Verification items for the finished model (mm, model axes). Face numbers are marked on the shaded views. A direction names the side the tool comes from. Round coordinates to 2 decimals unless told otherwise and drop trailing zeros. Write each loop counter-clockwise with the first axis right and the second up, starting at its lowest first coordinate (ties: lowest second). Pieces come first, ordered by that corner, then holes. Notation, with made-up numbers: (-15, -38.5) - (26, -38.5) arc R30 ccw to (26, -8.5) - close; hole circle Ø8 at (31, 19.25). An arc over 180 degrees is marked (long way). Answer as a JSON object with one key per item and string values.
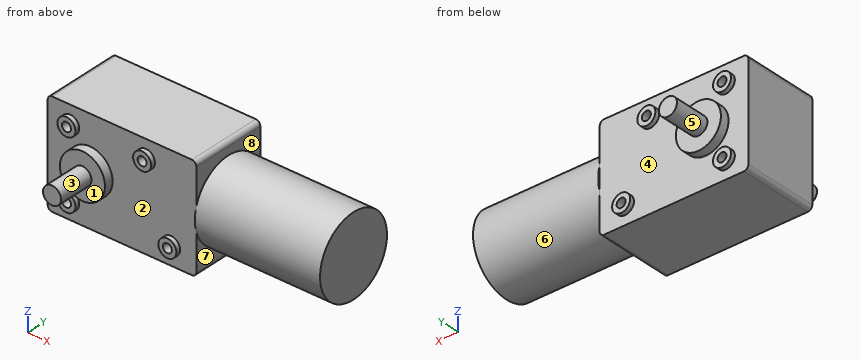
```python
from build123d import *

# Parameters (mm, degrees)
BOSS_EXTRUDE1_DEPTH = 21
SKETCH2_R           = 5
BOSS_EXTRUDE2_DEPTH = 2.5
SKETCH3_R           = 2.5
CUT_EXTRUDE1_DEPTH  = 6
SKETCH6_R           = 12.5
BOSS_EXTRUDE5_DEPTH = 5
SKETCH4_R           = 5
BOSS_EXTRUDE3_DEPTH = 20
SKETCH5_R           = 22
BOSS_EXTRUDE4_DEPTH = 69.5


with BuildPart() as part:
    # Sketch1 → Boss-Extrude1 (new, symmetric)
    with BuildSketch(Plane(origin=(0, 0, 0), x_dir=(1, 0, 0), z_dir=(0, 1, 0))):
        with BuildLine():
            Line((-38.75, -29), (38.75, -29))
            ThreePointArc((38.75, -29), (40.517766953, -28.267766953), (41.25, -26.5))
            Line((41.25, -26.5), (41.25, 26.5))
            ThreePointArc((41.25, 26.5), (40.517766953, 28.267766953), (38.75, 29))
            Line((38.75, 29), (-38.75, 29))
            ThreePointArc((-38.75, 29), (-40.517766953, 28.267766953), (-41.25, 26.5))
            Line((-41.25, 26.5), (-41.25, -26.5))
            ThreePointArc((-41.25, -26.5), (-40.517766953, -28.267766953), (-38.75, -29))
        make_face()
    extrude(amount=BOSS_EXTRUDE1_DEPTH, both=True)

    # Sketch2 → Boss-Extrude2 (add)
    with BuildSketch(Plane(origin=(0, 21, 0), x_dir=(1, 0, 0), z_dir=(0, 1, 0))):
        with Locations(Location((-28.75, 19, 0), (0, 0, 270))):
            Circle(SKETCH2_R)
        with Locations(Location((-28.75, -19, 0), (0, 0, 270))):
            Circle(SKETCH2_R)
        with Locations(Location((13.25, -19, 0), (0, 0, 270))):
            Circle(SKETCH2_R)
        with Locations(Location((27.25, 19, 0), (0, 0, 270))):
            Circle(SKETCH2_R)
    boss_extrude2 = extrude(amount=BOSS_EXTRUDE2_DEPTH)

    # Sketch3 → Cut-Extrude1 (cut)
    with BuildSketch(Plane(origin=(0, 23.5, 0), x_dir=(1, 0, 0), z_dir=(0, 1, 0))):
        with Locations(Location((-28.75, 19, 0), (0, 0, 270))):
            Circle(SKETCH3_R)
        with Locations(Location((27.25, 19, 0), (0, 0, 270))):
            Circle(SKETCH3_R)
        with Locations(Location((13.25, -19, 0), (0, 0, 270))):
            Circle(SKETCH3_R)
        with Locations(Location((-28.75, -19, 0), (0, 0, 270))):
            Circle(SKETCH3_R)
    cut_extrude1 = extrude(amount=-CUT_EXTRUDE1_DEPTH, mode=Mode.SUBTRACT)

    # Sketch6 → Boss-Extrude5 (add)
    with BuildSketch(Plane(origin=(0, 21, 0), x_dir=(1, 0, 0), z_dir=(0, 1, 0))):
        with Locations(Location((-17.75, 0, 0), (0, 0, 270))):
            Circle(SKETCH6_R)
    boss_extrude5 = extrude(amount=BOSS_EXTRUDE5_DEPTH)

    # Sketch4 → Boss-Extrude3 (add)
    with BuildSketch(Plane(origin=(0, 26, 0), x_dir=(1, 0, 0), z_dir=(0, 1, 0))):
        with Locations(Location((-17.75, 0, 0), (0, 0, 270))):
            Circle(SKETCH4_R)
    boss_extrude3 = extrude(amount=BOSS_EXTRUDE3_DEPTH)

    # Sketch5 → Boss-Extrude4 (add)
    with BuildSketch(Plane(origin=(41.25, 0, 0), x_dir=(0, 0, -1), z_dir=(1, 0, 0))):
        with Locations(Location((0, 0, 0), (0, 0, 107.341442803))):
            Circle(SKETCH5_R)
    extrude(amount=BOSS_EXTRUDE4_DEPTH)

    # Mirror2: Boss-Extrude2, Cut-Extrude1, Boss-Extrude5, Boss-Extrude3 across plane
    add(boss_extrude2.mirror(Plane.ZX))
    add(cut_extrude1.mirror(Plane.ZX), mode=Mode.SUBTRACT)
    add(boss_extrude5.mirror(Plane.ZX))
    add(boss_extrude3.mirror(Plane.ZX))


solid = part.part
```
Q1. Gauge pin test, flat ends, axial feed: P1, Ø1, axis at x = 81, z = -8.5, coming from the +Y side; P2, Ø12, axis at y = 35.5, z = -14, coming from the +X side; P3, Ø4, axis at x = 28, z = -18, coming from the +Y side; P4, Ø11, axis at x = -29.5, z = -19.5, coming from the -Y side. Record the tip position at first contact, or that the pin passes through.
Geometry check:
{"P1": "stops at y = 20.49", "P2": "passes through", "P3": "stops at y = 23.5", "P4": "stops at y = -23.5"}
Q2. Release check for a two-part mould opening along X. For the marked faces 1, 2, 3 and 4 record: released by +X, released by -X, zero draft, split by the parting line, or undercut.
Geometry check:
{"face 1": "zero draft", "face 2": "undercut", "face 3": "split by the parting line", "face 4": "undercut"}
Q3. Section check C-C, the plane z = 0. Record the cut outline in (x, y).
Geometry check:
{"outline": "(-41.25, -21) - (-30.25, -21) - (-30.25, -26) - (-22.75, -26) - (-22.75, -46) - (-12.75, -46) - (-12.75, -26) - (-5.25, -26) - (-5.25, -21) - (41.25, -21) - (41.25, -22) - (110.75, -22) - (110.75, 22) - (41.25, 22) - (41.25, 21) - (-5.25, 21) - (-5.25, 26) - (-12.75, 26) - (-12.75, 46) - (-22.75, 46) - (-22.75, 26) - (-30.25, 26) - (-30.25, 21) - (-41.25, 21) - close"}
Q4. Section check B-B, the plane y = 0. Record the cut outline in (x, z).
Geometry check:
{"outline": "(-41.25, -26.5) arc R2.5 ccw to (-38.75, -29) - (38.75, -29) arc R2.5 ccw to (41.25, -26.5) - (41.25, -22) - (110.75, -22) - (110.75, 22) - (41.25, 22) - (41.25, 26.5) arc R2.5 ccw to (38.75, 29) - (-38.75, 29) arc R2.5 ccw to (-41.25, 26.5) - close"}
Q5. Section check A-A, the plane x = -17.75. Record the cut outline in (y, z).
Geometry check:
{"outline": "(-46, -5) - (-26, -5) - (-26, -12.5) - (-21, -12.5) - (-21, -29) - (21, -29) - (21, -12.5) - (26, -12.5) - (26, -5) - (46, -5) - (46, 5) - (26, 5) - (26, 12.5) - (21, 12.5) - (21, 29) - (-21, 29) - (-21, 12.5) - (-26, 12.5) - (-26, 5) - (-46, 5) - close"}
Q6. Set-up check for the marked faces 5, 6, 7 and 8: record each of +Z, -Z, +X, -X, +Y, -Y from which the full face is reachable in a straight line by a thin tool's end or side.
Geometry check:
{"face 5": "+Y", "face 6": "+X", "face 7": "-Z, +X", "face 8": "+Z, +X"}
Q7. Section check D-D, the plane x = 27.25. Record the cut outline in (y, z).
Geometry check:
{"outline": "(-23.5, -24) - (-21, -24) - (-21, -29) - (21, -29) - (21, -24) - (23.5, -24) - (23.5, -21.5) - (17.5, -21.5) - (17.5, -16.5) - (23.5, -16.5) - (23.5, -14) - (21, -14) - (21, 29) - (-21, 29) - (-21, -14) - (-23.5, -14) - (-23.5, -16.5) - (-17.5, -16.5) - (-17.5, -21.5) - (-23.5, -21.5) - close"}
Q8. Material ranges on line 1 along X through (y, z) = (-20, 19); line 2 along X through (y, z) = (18.7, -19); line 3 along Z through (x, y) = (-28, -19), recorded low to high. Write a range as [from, to].
Geometry check:
{"line 1": "x = [-41.25, -31.25], [-26.25, 10.75], [15.75, 41.25]", "line 2": "x = [-41.25, -31.25], [-26.25, 24.75], [29.75, 41.25]", "line 3": "z = [-29, -21.38], [-16.62, 16.62], [21.38, 29]"}
